from build123d import *

# Parameters (mm, degrees)
BOSS_EXTRUDE1_DEPTH             = 241.3
BOSS_EXTRUDE1_DEPTH_BACK        = 198.12
SKETCH1_W                       = 13.97
SKETCH1_H                       = 12.758728324
BOSS_EXTRUDE2_REACH             = 243.485
SKETCH2_R                       = 9.525
BOSS_EXTRUDE2_DIRECTION_2_REACH = 243.485
SKETCH3_R                       = 4.191
CUT_EXTRUDE1_DEPTH              = 242.891662785
BOSS_EXTRUDE3_DEPTH             = 9.525
FILLET4_R                       = 25.4
FILLET5_R                       = 6.35
CUT_EXTRUDE2_DEPTH              = 294.005542012
CUT_EXTRUDE2_DEPTH_BACK         = 294.005542012
SKETCH6_R                       = 4.191


with BuildPart() as part:
    # Sketch1 → Boss-Extrude1 (new, two sides: drawn at the far end of the back side and taken through both)
    with BuildSketch(Plane.XY.offset(-BOSS_EXTRUDE1_DEPTH_BACK)):
        Rectangle(SKETCH1_W, SKETCH1_H)
    extrude(amount=BOSS_EXTRUDE1_DEPTH + BOSS_EXTRUDE1_DEPTH_BACK)

    # Boss-Extrude2: up to this face of the body (flat: up to its plane)
    boss_extrude2_end = Plane(part.part.faces().sort_by_distance((6.985, 0, 21.59))[0])
    # Sketch2 → Boss-Extrude2 (add, up to the picked face)
    with BuildSketch(Plane(origin=(0, 0, 0), x_dir=(0, 0, -1), z_dir=(1, 0, 0)), mode=Mode.PRIVATE) as boss_extrude2_sk1:
        with Locations((198.12, 0)):
            Circle(SKETCH2_R)
    boss_extrude2_tool1 = split(extrude(boss_extrude2_sk1.sketch, amount=BOSS_EXTRUDE2_REACH, mode=Mode.PRIVATE), bisect_by=boss_extrude2_end, keep=Keep.BOTH, mode=Mode.PRIVATE)
    add(boss_extrude2_tool1.solids().sort_by(Axis((0, 0, -198.12), (1, 0, 0)))[0])

    # Boss-Extrude2 direction 2: up to this face of the body (flat: up to its plane)
    boss_extrude2_direction_2_end = Plane(part.part.faces().sort_by_distance((-6.985, 0, 21.59))[0])
    # Sketch2 → Boss-Extrude2 direction 2 (add, up to the picked face)
    with BuildSketch(Plane(origin=(0, 0, 0), x_dir=(0, 0, -1), z_dir=(1, 0, 0)), mode=Mode.PRIVATE) as boss_extrude2_direction_2_sk1:
        with Locations((198.12, 0)):
            Circle(SKETCH2_R)
    boss_extrude2_direction_2_tool1 = split(extrude(boss_extrude2_direction_2_sk1.sketch, amount=-BOSS_EXTRUDE2_DIRECTION_2_REACH, mode=Mode.PRIVATE), bisect_by=boss_extrude2_direction_2_end, keep=Keep.BOTH, mode=Mode.PRIVATE)
    add(boss_extrude2_direction_2_tool1.solids().sort_by(Axis((0, 0, -198.12), (-1, 0, 0)))[0])

    # Sketch3 → Cut-Extrude1 (cut, through all)
    with BuildSketch(Plane(origin=(6.985, 0, 0), x_dir=(0, 0, -1), z_dir=(1, 0, 0))):
        with Locations((198.12, 0)):
            Circle(SKETCH3_R)
    extrude(amount=-CUT_EXTRUDE1_DEPTH, mode=Mode.SUBTRACT)

    # Sketch4 → Boss-Extrude3 (add, symmetric)
    with BuildSketch(Plane(origin=(0, 0, 0), x_dir=(1, 0, 0), z_dir=(0, 1, 0))):
        with BuildLine():
            Line((-6.985, -241.3), (-6.985, -292.1))
            Line((-6.985, -292.1), (-20.955, -292.1))
            Line((-20.955, -292.1), (-20.955, -238.518716551))
            ThreePointArc((-20.955, -238.518716551), (-17.180965419, -225.226169406), (-6.985, -215.9))
            Line((-6.985, -215.9), (-6.985, -241.3))
        make_face()
    boss_extrude3 = extrude(amount=BOSS_EXTRUDE3_DEPTH, both=True)

    # Mirror1: Boss-Extrude3 across plane
    add(boss_extrude3.mirror(Plane(origin=(0, 0, 0), x_dir=(0, 0, 1), z_dir=(1, 0, 0))))

    # Fillet4
    fillet4_edges = [part.edges().sort_by_distance(p)[0] for p in [
        (-6.985, 0, 215.9),
        (6.985, 0, 215.9),
    ]]
    fillet(fillet4_edges, radius=FILLET4_R)

    # Fillet5
    fillet5_edges = [part.edges().sort_by_distance(p)[0] for p in [
        (-13.97, -9.525, 292.1),
        (-13.97, 9.525, 292.1),
        (13.97, 9.525, 292.1),
        (13.97, -9.525, 292.1),
    ]]
    fillet(fillet5_edges, radius=FILLET5_R)

    # Sketch6 → Cut-Extrude2 (cut, two sides: drawn at the far end of the back side and taken through both)
    with BuildSketch(Plane(origin=(0, 0, 0), x_dir=(0, 0, -1), z_dir=(1, 0, 0)).offset(-CUT_EXTRUDE2_DEPTH_BACK)):
        with Locations((-279.32450026, 0)):
            Circle(SKETCH6_R)
    extrude(amount=CUT_EXTRUDE2_DEPTH + CUT_EXTRUDE2_DEPTH_BACK, mode=Mode.SUBTRACT)


solid = part.part
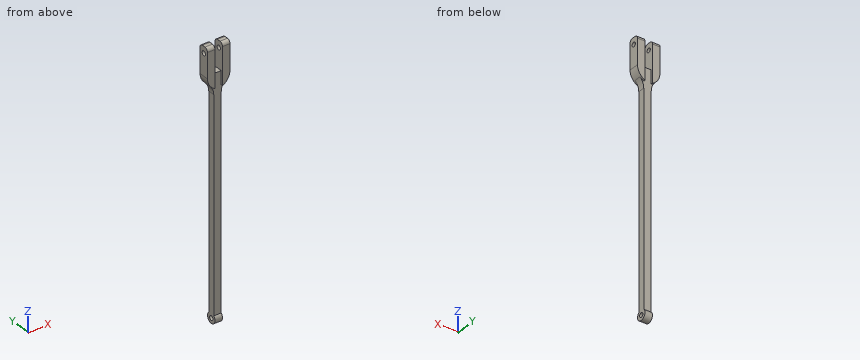
Geometry: final body of the model. Coordinates: model frame, mm. Give positions to 0.01 mm unless a question says otherwise; leave off trailing zeros. Loops run counter-clockwise (first coordinate to the right, second up) from the corner with the lowest first, then second, coordinate; pieces in that order, holes last. Notation, with made-up numbers: M -25,-20.75 L 15,-20.75 A8 cw 15,-15.75 Z; hole C -15,84 d10. An arc over 180 degrees is marked long. Put each result on its own line as item: value. Start each with the question number.
1) Cut plane A-A (y = 0). Output: boundary loops of the cut face in (x, z) (1 decimal).
2) Ray query, line 1 along Y through (x, z) = (-3.75, -198.12) (3 decimals); line 2 along X through (y, z) = (-4, -157) (3 decimals); line 3 along Y through (x, z) = (6, 40.5). Return the intervals inside material, ascending.
3) Cut plane B-B (z = -198.12). Output: boundary loops of the cut face in (x, y) (3 decimals), then the cut area to 3 significant figures.
4) Contact query for flat-ended pins moving along their axis: pin 1 (1 mm diameter, centred on x = -6, y = 4.5, fed in from -Z); pin 2 (6.5 mm diameter, centred on x = -2.5, y = 1.5, fed in from +Z); pin 3 (8 mm diameter, centred on x = 6.5, z = -42.5, fed in from -Y); pin 4 (5 mm diameter, centred on y = 0, z = 279.32, fed in from +X). Output: stop coordinate, or through.
5) Cut plane C-C (z = 71). Output: boundary loops of the cut face in (x, y) (3 decimals).
Verdict:
1. outline: M -21,238.5 A25.3 ccw -14,221.1 A25.4 cw -7,203.6 L -7,-193.9 L 7,-193.9 L 7,203.6 A25.4 cw 14,221.1 A25.3 ccw 21,238.5 L 21,275.1 L 7,275.1 L 7,241.3 L -7,241.3 L -7,275.1 L -21,275.1 Z; M -21,283.5 L -7,283.5 L -7,292.1 L -21,292.1 Z; M -7,-207.6 L 7,-207.6 L 7,-202.3 L -7,-202.3 Z; M 7,283.5 L 21,283.5 L 21,292.1 L 7,292.1 Z
2. line 1: -9.525 to -4.191, 4.191 to 9.525
2. line 2: -6.985 to 6.985
2. line 3: -6.38 to 6.38
3. outline: M -6.985,-9.525 L 6.985,-9.525 L 6.985,-4.191 L -6.985,-4.191 Z; M -6.985,4.191 L 6.985,4.191 L 6.985,9.525 L -6.985,9.525 Z
3. area: 149 mm2
4. pin 1: z = -206.76
4. pin 2: z = 241.3
4. pin 3: y = -6.38
4. pin 4: through
5. outline: M -6.985,-6.379 L 6.985,-6.379 L 6.985,6.379 L -6.985,6.379 Z
